For this review, take the finished solid that the model builds, in its own axes (mm). A direction names the side the tool comes from. Round coordinates to 2 decimals unless told otherwise and drop trailing zeros. Loops run counter-clockwise (first coordinate to the right, second up) from the corner with the lowest first, then second, coordinate; pieces in that order, holes last.
1. Clearance check with flat-ended pins moving along their axes: pin 1 Ø4 at (x, y) = (0, -4) entering from -Z; pin 2 Ø4 at (x, y) = (-4.5, 9.5) entering from -Z; pin 3 Ø1 at (y, z) = (-13.5, 3) entering from +X. State where each tip first meets the part, or that it passes through.
2. Draft analysis for pull direction X (two halves, no side actions). For faces 1 (the cylindrical face through (-13.175, 12.081, 2.465)), 2 (the flat face through (4, -4, 5)), 3 (the cylindrical face through (-0.33, 13.65, -6.97)), state which applies: released by +X, released by -X, zero draft, split by the parting line, or undercut.
3. Consider section A-A on y = 0. State the section outline as (x, z) points (3 decimals), then the cut area to 3 significant figures.
4. To check wall thickness, follow line 1 along Y through (x, z) = (0, 2.8) (3 decimals); line 2 along Z through (x, y) = (-13.5, 9); line 3 along Z through (x, y) = (-2, 14). State the ranges of each line that lie inside material, in increasing order.
5. Consider section B-B on x = 0. State the section outline as (y, z) points (1 decimal), then the cut area to 3 significant figures.
6. Consider section D-D on z = -6.5. State the section outline as (x, y) points, then the cut area to 3 significant figures.
7. Tool access review of faces 4 (the flat face through (0, 15, -5)), 5 (the cylindrical face through (-0.59, 4.46, 2.46)): name each direction out of +Z, -Z, +X, -X, +Y, -Y from which nothing blocks a thin tool from reaching the whole face with its end or side.
8. Consider section C-C on y = 4. State the section outline as (x, z) points.
from build123d import *

# Parameters (mm, degrees)
F0_R     = 17.875
F0_R_2   = 4.5
F1_DEPTH = 5
F2_R     = 3.6875
F3_DEPTH = 10
F4_R     = 2.5
F4_R_2   = 1.5
F5_DEPTH = 4
F6_R     = 0.842662
F7_DEPTH = 25


with BuildPart() as f1:
    # F0 (on Top) → F1 (new body)
    with BuildSketch(Plane.XY):
        Circle(F0_R)
        Circle(F0_R_2, mode=Mode.SUBTRACT)
    extrude(amount=F1_DEPTH)

    # F2 (on face) → F3 (join)
    with BuildSketch(Plane.XY.offset(5)):
        with Locations((0, 12.1875)):
            Circle(F2_R)
    extrude(amount=-F3_DEPTH)

    # F4 (on face) → F5 (join)
    with BuildSketch(Plane(origin=(0, 0, -5), x_dir=(1, 0, 0), z_dir=(0, 0, -1))):
        with Locations((0, -12.1875)):
            Circle(F4_R)
        with Locations((0, -12.1875)):
            Circle(F4_R_2, mode=Mode.SUBTRACT)
    extrude(amount=F5_DEPTH)

    # F6 (on Top) → F7 (cut)
    with BuildSketch(Plane.XY):
        with Locations((-10.189319, 10.732485)):
            Circle(F6_R)
    extrude(amount=F7_DEPTH, mode=Mode.SUBTRACT)


solid = f1.part
Resolved:
1. pin 1: stops at z = 0
1. pin 2: stops at z = -5
1. pin 3: stops at x = 12.27
2. face 1: split by the parting line
2. face 2: zero draft
2. face 3: undercut
3. outline: (-17.875, 0) - (-4.5, 0) - (-4.5, 5) - (-17.875, 5) - close; (4.5, 0) - (17.875, 0) - (17.875, 5) - (4.5, 5) - close
3. area: 134 mm2
4. line 1: y = -17.875 to -4.5, 4.5 to 17.875
4. line 2: z = 0 to 5
4. line 3: z = -5 to 5
5. outline: (-17.9, 0) - (-4.5, 0) - (-4.5, 5) - (-17.9, 5) - close; (4.5, 0) - (8.5, 0) - (8.5, -5) - (9.7, -5) - (9.7, -9) - (10.7, -9) - (10.7, -5) - (13.7, -5) - (13.7, -9) - (14.7, -9) - (14.7, -5) - (15.9, -5) - (15.9, 0) - (17.9, 0) - (17.9, 5) - (4.5, 5) - close
5. area: 179 mm2
6. outline: circle Ø5 at (0, 12.19); hole circle Ø3 at (0, 12.19)
6. area: 12.6 mm2
7. face 4: -Z
7. face 5: +Z, -Z
8. outline: (-17.42, 0) - (-2.06, 0) - (-2.06, 5) - (-17.42, 5) - close; (2.06, 0) - (17.42, 0) - (17.42, 5) - (2.06, 5) - close
